Work out the finished part from the listing and answer in its coordinate system (mm). Give positions to 0.01 mm unless a question says otherwise; leave off trailing zeros. Order: outer loops, then holes, each group sorted by start corner. A loop starts at its lowest first (then second) coordinate and runs counter-clockwise, first axis right, second up. Notation, with made-up numbers: (-30, -34) -> (-22, -34) arc R15 ccw to (-22, -8) -> close; hole circle Ø8 at (-24, 7.5). An arc over 180 degrees is marked (long way). Use a Markdown table: item, result. Add a question column.
```python
from build123d import *

# Parameters (mm, degrees)
SKETCH1_W                       = 192
SKETCH1_H                       = 25
BOSS_EXTRUDE1_DEPTH             = 2.4
SKETCH2_R                       = 1.4
CUT_EXTRUDE1_DEPTH              = 194.635637216
SKETCH3_W                       = 5
SKETCH3_H                       = 40
BOSS_EXTRUDE2_DEPTH             = 30
BOSS_EXTRUDE2_DIRECTION_2_REACH = 195.636
SKETCH4_R                       = 3.15
CUT_EXTRUDE2_DEPTH              = 30
SKETCH8_W                       = 10
SKETCH8_H                       = 2
BOSS_EXTRUDE4_DEPTH             = 187
SKETCH9_W                       = 20
SKETCH9_H                       = 13.857334598
CUT_EXTRUDE4_DEPTH              = 199.403628999
CHAMFER5_SIZE                   = 6


with BuildPart() as part:
    # Sketch1 → Boss-Extrude1 (new body)
    with BuildSketch(Plane.XY):
        with Locations((96, 12.5)):
            Rectangle(SKETCH1_W, SKETCH1_H)
    extrude(amount=BOSS_EXTRUDE1_DEPTH)

    # Sketch2 → Cut-Extrude1 (cut, through all)
    with BuildSketch(Plane.XY.offset(2.4)):
        with Locations((87, 20.5)):
            Circle(SKETCH2_R)
        with Locations(Location((57, 20.5, 0), (0, 0, 180))):
            Circle(SKETCH2_R)
        with Locations(Location((152, 20.5, 0), (0, 0, 180))):
            Circle(SKETCH2_R)
        with Locations((182, 20.5)):
            Circle(SKETCH2_R)
        Polygon((177, 25), (172, 13), (162, 13), (157, 25), align=None)
        Polygon((82, 25), (77, 13), (67, 13), (62, 25), align=None)
    extrude(amount=-CUT_EXTRUDE1_DEPTH, mode=Mode.SUBTRACT)

    # Sketch3 → Boss-Extrude2 (add)
    with BuildSketch(Plane(origin=(0, 0, 0), x_dir=(-1, 0, 0), z_dir=(0, 0, -1))):
        with Locations((-2.5, 5)):
            Rectangle(SKETCH3_W, SKETCH3_H)
    extrude(amount=BOSS_EXTRUDE2_DEPTH)

    # Boss-Extrude2 direction 2: up to this face of the body (flat: up to its plane)
    boss_extrude2_direction_2_end = Plane(part.part.faces().sort_by_distance((93.952876609, 11.871051408, 2.4))[0])
    # Sketch3 → Boss-Extrude2 direction 2 (add, up to the picked face)
    with BuildSketch(Plane(origin=(0, 0, 0), x_dir=(-1, 0, 0), z_dir=(0, 0, -1)), mode=Mode.PRIVATE) as boss_extrude2_direction_2_sk1:
        with Locations((-2.5, 5)):
            Rectangle(SKETCH3_W, SKETCH3_H)
    boss_extrude2_direction_2_tool1 = split(extrude(boss_extrude2_direction_2_sk1.sketch, amount=-BOSS_EXTRUDE2_DIRECTION_2_REACH, mode=Mode.PRIVATE), bisect_by=boss_extrude2_direction_2_end, keep=Keep.BOTH, mode=Mode.PRIVATE)
    add(boss_extrude2_direction_2_tool1.solids().sort_by(Axis((2.5, 5, 0), (0, 0, 1)))[0])

    # Sketch4 → Cut-Extrude2 (cut)
    with BuildSketch(Plane.ZY):
        with Locations((-13.6, 16)):
            Circle(SKETCH4_R)
        with Locations((-13.6, -6)):
            Circle(SKETCH4_R)
    extrude(amount=-CUT_EXTRUDE2_DEPTH, mode=Mode.SUBTRACT)

    # Sketch8 → Boss-Extrude4 (add)
    with BuildSketch(Plane(origin=(5, 0, 0), x_dir=(0, 0, -1), z_dir=(1, 0, 0))):
        with Locations((5, 5)):
            Rectangle(SKETCH8_W, SKETCH8_H)
    extrude(amount=BOSS_EXTRUDE4_DEPTH)

    # Sketch9 → Cut-Extrude4 (cut, through all)
    with BuildSketch(Plane(origin=(0, 25, 0), x_dir=(1, 0, 0), z_dir=(0, 1, 0))):
        with Locations((72, 6.928667299)):
            Rectangle(SKETCH9_W, SKETCH9_H)
        with Locations((167, 6.928667299)):
            Rectangle(SKETCH9_W, SKETCH9_H)
    extrude(amount=-CUT_EXTRUDE4_DEPTH, mode=Mode.SUBTRACT)

    # Chamfer5
    chamfer5_edges = [part.edges().sort_by_distance(p)[0] for p in [
        (62, 5, -10),
        (82, 5, -10),
        (157, 5, -10),
        (177, 5, -10),
        (192, 5, -10),
    ]]
    chamfer(chamfer5_edges, length=CHAMFER5_SIZE)


solid = part.part
```
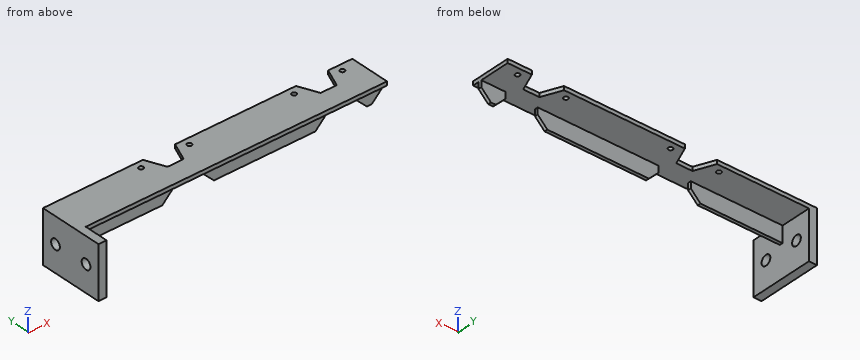
1) The part is cut by section A-A, the plane y = 16. Determine the outline of the cut face in (x, z), then the cut area to 3 significant figures.
2) Straight lines are drawn through the part: line 1 (Y direction, x = 1.05, z = -13.6); line 2 (Y direction, x = 87, z = 1.6); line 3 (Z direction, x = 29, y = 20). For each, find the intervals that lie inside material, in ascending order.
3) The part is cut by section C-C, the plane y = -6. Determine the outline of the cut face in (x, z), then the cut area to 4 significant figures.
4) Flat-ended cylindrical pins translate along their axes: pin 1 (12 mm diameter, centred on x = 111.5, z = -14, fed in from -Y); pin 2 (4.5 mm diameter, centred on x = 182, y = 20.5, fed in from -Z); pin 3 (4 mm diameter, centred on y = -0.5, z = -21.5, fed in from +X); pin 4 (6 mm diameter, centred on x = 50, z = -15.5, fed in from -Y). Find the tip coordinate at first contact, or state that the pin passes through.
5) The part is cut by section B-B, the plane z = -13.6. Determine the outline of the cut face in (x, y).
6) The part is cut by section D-D, the plane x = 51. Determine the outline of the cut face in (y, z).
A:
| question | item | result |
|---|---|---|
| 1 | outline | (0, -30) -> (5, -30) -> (5, -16.75) -> (0, -16.75) -> close; (0, -10.45) -> (5, -10.45) -> (5, 0) -> (65.75, 0) -> (65.75, 2.4) -> (0, 2.4) -> close; (78.25, 0) -> (160.75, 0) -> (160.75, 2.4) -> (78.25, 2.4) -> close; (173.25, 0) -> (192, 0) -> (192, 2.4) -> (173.25, 2.4) -> close |
| 1 | area | 519 mm^2 |
| 2 | line 1 | -15 to -9.15, -2.85 to 12.85, 19.15 to 25 |
| 2 | line 2 | 0 to 19.1, 21.9 to 25 |
| 2 | line 3 | 0 to 2.4 |
| 3 | outline | (0, -30) -> (5, -30) -> (5, -16.75) -> (0, -16.75) -> close; (0, -10.45) -> (5, -10.45) -> (5, 2.4) -> (0, 2.4) -> close |
| 3 | area | 130.5 mm^2 |
| 4 | pin 1 | y = 4 |
| 4 | pin 2 | z = 0 |
| 4 | pin 3 | x = 5 |
| 4 | pin 4 | through |
| 5 | outline | (0, -15) -> (5, -15) -> (5, -9.15) -> (0, -9.15) -> close; (0, -2.85) -> (5, -2.85) -> (5, 12.85) -> (0, 12.85) -> close; (0, 19.15) -> (5, 19.15) -> (5, 25) -> (0, 25) -> close |
| 6 | outline | (0, 0) -> (4, 0) -> (4, -10) -> (6, -10) -> (6, 0) -> (25, 0) -> (25, 2.4) -> (0, 2.4) -> close |
